```python
from build123d import *
from build123d.topology import SkipClean

# Parameters (mm, degrees)
BOSS_EXTRUDE1_DEPTH = 20
SKETCH2_R           = 5
BOSS_EXTRUDE2_DEPTH = 41
CUT_EXTRUDE1_DEPTH  = 41
SKETCH4_R           = 2.5
CUT_EXTRUDE2_DEPTH  = 50.809637702
FILLET1_R           = 2
SKETCH5_R           = 10
BOSS_EXTRUDE3_DEPTH = 15
CUT_EXTRUDE3_DEPTH  = 5
CHAMFER1_SIZE       = 2


with BuildPart() as part:
    # Sketch1 → Boss-Extrude1 (new body)
    with BuildSketch(Plane(origin=(0, 0, 0), x_dir=(1, 0, 0), z_dir=(0, 1, 0))):
        with BuildLine():
            ThreePointArc((0.5, -14.991664351), (14.997915943, 0.250034739), (0, 15))
            Line((0, 15), (-30, 15))
            Line((-30, 15), (-30, -15))
            Line((-30, -15), (-0.5, -15))
            Line((-0.5, -15), (-0.5, -9.987492178))
            ThreePointArc((-0.5, -9.987492178), (0, 10), (0.5, -9.987492178))
            Line((0.5, -9.987492178), (0.5, -14.991664351))
        make_face()
    extrude(amount=BOSS_EXTRUDE1_DEPTH)

    # Sketch2 → Boss-Extrude2 (add)
    with BuildSketch(Plane.ZY.offset(30)):
        with Locations(Location((15, 10, 0), (0, 0, 270))):
            Circle(SKETCH2_R)
    extrude(amount=-BOSS_EXTRUDE2_DEPTH)

    # Sketch3 → Cut-Extrude1 (cut)
    with BuildSketch(Plane(origin=(0, 20, 0), x_dir=(1, 0, 0), z_dir=(0, 1, 0))):
        Polygon((-0.5, -15), (-0.5, -9.987492178), (0.5, -9.987492178), (0.5, -14.991664351), (0.5, -20), (-0.5, -20), align=None)
    extrude(amount=-CUT_EXTRUDE1_DEPTH, mode=Mode.SUBTRACT)

    # Sketch4 → Cut-Extrude2 (cut, through all)
    with BuildSketch(Plane(origin=(11, 0, 0), x_dir=(0, 0, -1), z_dir=(1, 0, 0))):
        with Locations((-15, 10)):
            Circle(SKETCH4_R)
    extrude(amount=-CUT_EXTRUDE2_DEPTH, mode=Mode.SUBTRACT)

    # Fillet1
    fillet1_edges = [part.edges().sort_by_distance(p)[0] for p in [
        (-15, 0, -15),
        (14.997915943, 0, -0.250034739),
        (-15, 20, -15),
        (-15.25, 20, 15),
        (14.997915943, 20, -0.250034739),
        (-15.25, 0, 15),
    ]]
    fillet(fillet1_edges, radius=FILLET1_R)

    # Sketch5 → Boss-Extrude3 (add)
    with BuildSketch(Plane.ZY.offset(30)):
        with Locations(Location((0, 10, 0), (0, 0, 270))):
            Circle(SKETCH5_R)
    extrude(amount=BOSS_EXTRUDE3_DEPTH)

    # Sketch6 → Cut-Extrude3 (cut)
    with SkipClean():  # the faces are left unmerged after this step: merging them gives an invalid solid
        with BuildSketch(Plane.ZY.offset(30)):
            with BuildLine():
                ThreePointArc((0, 0), (-10, 10), (0, 20))
                Line((0, 20), (-13, 20))
                ThreePointArc((-13, 20), (-14.414213562, 19.414213562), (-15, 18))
                Line((-15, 18), (-15, 2))
                ThreePointArc((-15, 2), (-14.414213562, 0.585786438), (-13, 0))
                Line((-13, 0), (0, 0))
            make_face()
            with BuildLine():
                Line((13, 20), (0, 20))
                ThreePointArc((0, 20), (10, 10), (0, 0))
                Line((0, 0), (13, 0))
                ThreePointArc((13, 0), (14.414213562, 0.585786438), (15, 2))
                Line((15, 2), (15, 5))
                ThreePointArc((15, 5), (20, 10), (15, 15))
                Line((15, 15), (15, 18))
                ThreePointArc((15, 18), (14.414213562, 19.414213562), (13, 20))
            make_face()
        extrude(amount=-CUT_EXTRUDE3_DEPTH, mode=Mode.SUBTRACT)

    # Chamfer1
    chamfer1_edges = [part.edges().sort_by_distance(p)[0] for p in [
        (-45, 20, 0),
    ]]
    chamfer(chamfer1_edges, length=CHAMFER1_SIZE)


solid = part.part
```
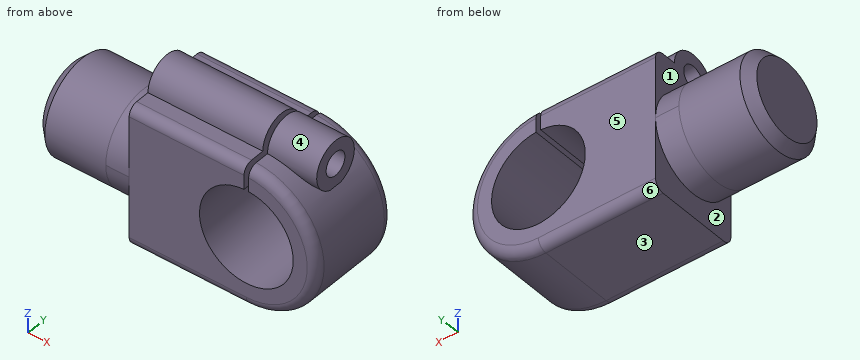
The listing builds one solid part. Answer for the finished solid, in the listing's coordinates (mm). Face numbers are marked on the shaded views. A direction names the side the tool comes from. Give positions to 0.01 mm unless a question says otherwise; leave off trailing zeros. Loops run counter-clockwise (first coordinate to the right, second up) from the corner with the lowest first, then second, coordinate; pieces in that order, holes last. Notation, with made-up numbers: (33, 41.25) - (73, 41.25) arc R33 cw to (73, 70.25) - close; hole circle Ø6 at (-40, 55). An arc over 180 degrees is marked (long way). Return JSON: item names as keys, results as strings. Group by question number.
1. Straight lines are drawn through the part: line 1 (Y direction, x = 7, z = 15); line 2 (Z direction, x = -3.5, y = 11); line 3 (Z direction, x = -23, y = 9.25). For each, find the intervals that lie inside material, in ascending order. Write a range as [from, to].
2. Given pin 1 Ø16 at (x, z) = (0, 0) entering from -Y; pin 2 Ø6 at (y, z) = (10, 15) entering from -X; pin 3 Ø1.5 at (x, y) = (-9, 16) entering from +Z; pin 4 Ø8 at (y, z) = (10.5, 13) entering from -X, each flat-ended and moving along its own axis, determine where each tip first touches the part or whether it passes through.
3. Find section B-B (y = 10). Write down the section's boundary in (x, z).
4. Find section A-A (x = -4). Write down the section's boundary in (y, z).
5. Determine the mould class of the marked faces 4, 5 and 6 for opening direction Z: pulls with the +Z half, pulls with the -Z half, needs draft (parallel to the pull), parting line crosses it, or undercut.
6. Which of the six approach directions +Z, -Z, +X, -X, +Y, -Y give full straight-line access (tool end or side, diameter ignored) to the marked faces 1, 2 and 3?
Verdict:
{
 "1": {"line 1": "y = [5, 7.5], [12.5, 15]", "line 2": "z = [-15, -9.37], [9.37, 12.71], [17.29, 19.9]", "line 3": "z = [-15, 12.62], [17.38, 19.94]"},
 "2": {"pin 1": "passes through", "pin 2": "stops at x = -25", "pin 3": "stops at z = 15", "pin 4": "stops at x = -43.99"},
 "3": {"outline": "(-45, -8) - (-43, -10) - (-25, -10) - (-25, -15) - (0, -15) arc R15 ccw to (11, 10.2) - (11, 12.5) - (0.5, 12.5) - (0.5, 9.99) arc R10 cw (long way) to (-0.5, 9.99) - (-0.5, 12.5) - (-25, 12.5) - (-25, 10) - (-43, 10) - (-45, 8) - close; (-25, 17.5) - (-0.5, 17.5) - (-0.5, 20) - (-25, 20) - close; (0.5, 17.5) - (11, 17.5) - (11, 20) - (0.5, 20) - close"},
 "4": {"outline": "(0, -13) arc R2 ccw to (2, -15) - (18, -15) arc R2 ccw to (20, -13) - (20, -9.17) - (0, -9.17) - close; (0, 9.17) - (20, 9.17) - (20, 13) arc R2 ccw to (18, 15) - (15, 15) arc R5 ccw to (5, 15) - (2, 15) arc R2 ccw to (0, 13) - close; hole circle Ø5 at (10, 15)"},
 "5": {"face 4": "undercut", "face 5": "needs draft", "face 6": "pulls with the -Z half"},
 "6": {"face 1": "+Z, -X", "face 2": "-Z, -X", "face 3": "-Z, +X, -X, +Y, -Y"}
}
